from build123d import *

# Parameters (mm, degrees)
F0_W          = 20
F0_H          = 20
F1_DEPTH      = 10
F1_DEPTH_BACK = 10
F2_R          = 8
F2_R_2        = 7
F3_DEPTH      = 30
F4_W          = 5
F4_H          = 5
F5_DEPTH      = 30
F9_COUNT      = 2
F9_ANGLE      = 90
F10_COUNT     = 2
F10_ANGLE     = 90


with BuildPart() as f1:
    # F0 (on Top) → F1 (new body, two sides)
    with BuildSketch(Plane.XY) as f1_sk:
        Rectangle(F0_W, F0_H)
    extrude(amount=-F1_DEPTH)
    extrude(f1_sk.sketch, amount=F1_DEPTH_BACK)

    # F2 (on face) → F3 (join)
    with BuildSketch(Plane.XY.offset(10)):
        Circle(F2_R)
        Circle(F2_R_2, mode=Mode.SUBTRACT)
    extrude(amount=F3_DEPTH)

    # F4 (on face) → F5 (join)
    with BuildSketch(Plane.XY.offset(10)):
        Rectangle(F4_W, F4_H)
    extrude(amount=F5_DEPTH)

    # F6 (on Front) → F7 (revolve, cut)
    with BuildSketch(Plane.XZ):
        Polygon((0, 39.9759672582), (0.0436493601, 39.9563506399), (6.35, 33.65), (6.35, 40), (0, 40), align=None)
    revolve(axis=Axis((0, 0, 38.1132610887), (0, 0, -1)), mode=Mode.SUBTRACT)

    # F9: F1 ×2 about axis
    f9_axis = Axis((7.9106530175, 0, 0), (-1, 0, 0))


with BuildPart() as f1_1:
    add(f1.part)
    for i in range(1, F9_COUNT):
        add(f1.part.rotate(f9_axis, i * F9_ANGLE / (F9_COUNT - 1)))

    # F10: F1 ×2 about axis
    f10_axis = Axis((0, 10, 0), (0, -1, 0))


with BuildPart() as f1_2:
    add(f1_1.part)
    for i in range(1, F10_COUNT):
        add(f1_1.part.rotate(f10_axis, i * F10_ANGLE / (F10_COUNT - 1)))


solid = f1_2.part
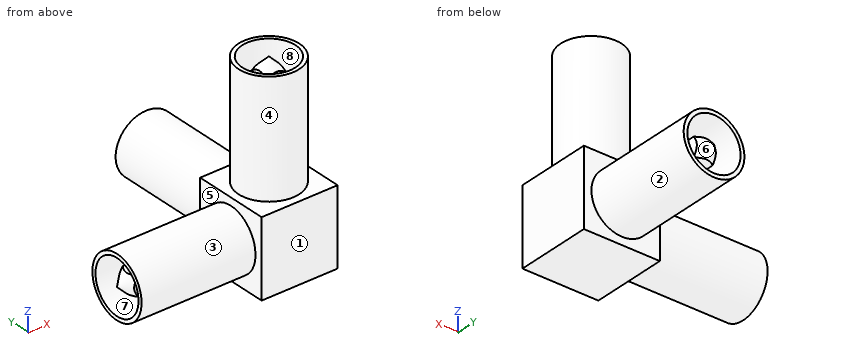
Could you check a few things on this model? Use its own coordinates, in mm. Face numbers are marked on the shaded views. A direction names the side the tool comes from. Give positions to 0.01 mm unless a question says otherwise; leave off trailing zeros. Order: outer loops, then holes, each group sorted by start corner. A loop starts at its lowest first (then second) coordinate and runs counter-clockwise, first axis right, second up. Notation, with made-up numbers: (55.25, 37) - (82.25, 37) arc R35 cw to (82.25, 76) - close; hole circle Ø1 at (-29.5, -1). An arc over 180 degrees is marked (long way). One line per item, written item: value. Start each with the question number.
1. Imagine slicing it at A-A on y = 25.5. List the corners of the cut face in (x, z) for me, plus the area to 3 significant figures.
2. For the marked faces 1, 2, 3 and 4, which set-ups out of +Z, -Z, +X, -X, +Y, -Y let a thin tool reach every point of the face, with its end or its side?
3. Imagine slicing it at C-C on x = 4. List the corners of the cut face in (y, z) for me, plus the area to 3 significant figures.
4. Thinking about a two-plate mould opening in X: for the marked faces 5, 6, 7 and 8, which applies, +X half, -X half, draft (parallel to the pull), parting line (faces both ways), or undercut?
5. If I drill on probe 1 along Y at (x, z) = (-20, 0); probe 2 along Z at (x, y) = (0.5, 19); probe 3 along X at (y, z) = (-2, 11), over which ranges is the centre line in solid material (lowest first)?
6. For P1, Ø4, axis at x = -0.5, y = 26, coming from the +Z side; P2, Ø5.5, axis at x = -1, z = 30, coming from the -Y side; P3, Ø2.5, axis at y = -1, z = 18, coming from the -X side; P4, Ø15.5, axis at x = 1, z = -3, coming from the +Y side, each with a flat end and sliding along its axis, tell me the tip position at first contact or that it passes through.
7. Imagine slicing it at D-D on y = 4.5. List the corners of the cut face in (x, z) for me.
Values:
1. outline: circle Ø16 at (0, 0); (-2.5, -2.5) - (2.5, -2.5) - (2.5, 2.5) - (-2.5, 2.5) - close; hole circle Ø14 at (0, 0)
1. area: 72.1 mm²
2. face 1: +Z, -Z, +X, -X, -Y
2. face 2: +Y
2. face 3: -X
2. face 4: +Z
3. outline: (-10, -10) - (10, -10) - (10, -6.93) - (40, -6.93) - (40, -5.74) - (10, -5.74) - (10, 5.74) - (40, 5.74) - (40, 6.93) - (10, 6.93) - (10, 10) - (6.93, 10) - (6.93, 40) - (5.74, 40) - (5.74, 10) - (-5.74, 10) - (-5.74, 40) - (-6.93, 40) - (-6.93, 10) - (-10, 10) - close
3. area: 542 mm²
4. face 5: -X half
4. face 6: undercut
4. face 7: draft
4. face 8: undercut
5. probe 1: -8 to -7, -2.5 to 2.5, 7 to 8
5. probe 2: -7.98 to -6.98, -2.5 to 2.5, 6.98 to 7.98
5. probe 3: -7.75 to -6.71, -2.5 to 2.5, 6.71 to 7.75
6. P1: z = 8
6. P2: y = -8
6. P3: x = -8
6. P4: y = 40
7. outline: (-40, -6.61) - (-10, -6.61) - (-10, -10) - (10, -10) - (10, 10) - (6.61, 10) - (6.61, 40) - (5.36, 40) - (5.36, 10) - (-5.36, 10) - (-5.36, 40) - (-6.61, 40) - (-6.61, 10) - (-10, 10) - (-10, 6.61) - (-40, 6.61) - (-40, 5.36) - (-10, 5.36) - (-10, -5.36) - (-40, -5.36) - close
